Job drawing, mm, ordinate dimensions from the low corner. One solid piece. Give positions to 0.01 mm unless a question says otherwise; leave off trailing zeros. Order: outer loops, then holes, each group sorted by start corner. A loop starts at its lowest first (then second) coordinate and runs counter-clockwise, first axis right, second up.
1. Drop flat-ended pins along their axis: pin 1 Ø1.2 at (y, z) = (21, 2) entering from -X; pin 2 Ø2 at (y, z) = (17, 1) entering from -X. Give the stop position or say it passes through.
2. Probe line 1 (Y direction, x = 12.5, z = 2.45); line 2 (X direction, y = 23.25, z = 1.55); line 3 (X direction, y = 14, z = 2.7). List the from-to ranges inside material, lowest first.
3. Slice it at A-A on z = 1.6. List the corners of the cut face in (x, y).
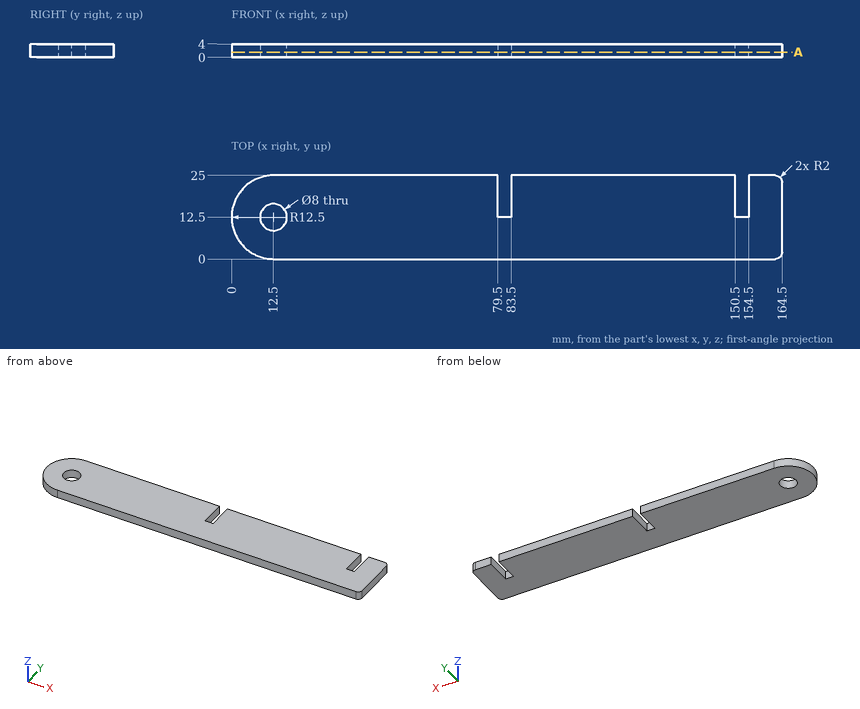
Data:
1. pin 1: stops at x = 2.81
1. pin 2: stops at x = 0.5
2. line 1: y = 0 to 8.5, 16.5 to 25
2. line 2: x = 6.12 to 79.5, 83.5 to 150.5, 154.5 to 164.48
2. line 3: x = 0.09 to 8.79, 16.21 to 79.5, 83.5 to 150.5, 154.5 to 164.5
3. outline: (12.5, 0) - (162.5, 0) arc R2 ccw to (164.5, 2) - (164.5, 23) arc R2 ccw to (162.5, 25) - (154.5, 25) - (154.5, 12.5) - (150.5, 12.5) - (150.5, 25) - (83.5, 25) - (83.5, 12.5) - (79.5, 12.5) - (79.5, 25) - (12.5, 25) arc R12.5 ccw to start; hole circle Ø8 at (12.5, 12.5)
